Design review of the part built by this model. Coordinates are the model's own, in mm. A direction names the side the tool comes from. Coordinates: 2 decimals unless noted, no trailing zeros. Write each loop counter-clockwise with the first axis right and the second up, starting at its lowest first coordinate (ties: lowest second). Pieces come first, ordered by that corner, then holes. Notation, with made-up numbers: (2.25, 16.25) - (21.25, 16.25) arc R14 ccw to (21.25, 39.25) - close; hole circle Ø6 at (-39, 49.5). An arc over 180 degrees is marked (long way). Use a Markdown table: item, result.
from build123d import *

# Parameters (mm, degrees)
SKETCH1_W = 40
SKETCH1_H = 1
SKETCH2_W = 3
SKETCH2_H = 6


with BuildPart() as part:
    # Sketch1 → Base-Revolve (revolve)
    with BuildSketch(Plane.XY, mode=Mode.PRIVATE) as base_revolve_sk:
        with Locations((0, 4.5)):
            Rectangle(SKETCH1_W, SKETCH1_H)
    revolve(base_revolve_sk.sketch.rotate(Axis((-20, 0, 0), (1, 0, 0)), 90), axis=Axis((-20, 0, 0), (1, 0, 0)))

    # Sketch2 → Cut-for-GripLength (revolve, cut)
    with BuildSketch(Plane.XY):
        with Locations((-18.5, 3)):
            Rectangle(SKETCH2_W, SKETCH2_H)
        with Locations((18.5, 3)):
            Rectangle(SKETCH2_W, SKETCH2_H)
    revolve(axis=Axis((-30, 0, 0), (1, 0, 0)), mode=Mode.SUBTRACT)

    # Sketch3 → HeadTypeA (revolve)
    with BuildSketch(Plane.XY, mode=Mode.PRIVATE) as headtypea_sk:
        with BuildLine():
            Line((-19, 6), (-19, 7.5))
            Line((-19, 7.5), (-18, 7.5))
            Line((-18, 7.5), (-18, 6))
            ThreePointArc((-18, 6), (-17.707106781, 5.292893219), (-17, 5))
            Line((-17, 5), (-17, 4))
            ThreePointArc((-17, 4), (-18.414213562, 4.585786438), (-19, 6))
        make_face()
        with BuildLine():
            Line((19, 6), (19, 7.5))
            Line((19, 7.5), (18, 7.5))
            Line((18, 7.5), (18, 6))
            ThreePointArc((18, 6), (17.707106781, 5.292893219), (17, 5))
            Line((17, 5), (17, 4))
            ThreePointArc((17, 4), (18.414213562, 4.585786438), (19, 6))
        make_face()
    revolve(headtypea_sk.sketch.rotate(Axis((-20, 0, 0), (1, 0, 0)), 90), axis=Axis((-20, 0, 0), (1, 0, 0)))


solid = part.part
(1) Draft analysis for pull direction Z (two halves, no side actions). For faces 3 (the cylindrical face through (0.238, 3.905, -0.867)), 4 (the cylindrical face through (-18.493, -6.324, 4.032)), 5 (the flat face through (18, -6, 2)), state which applies: +Z half, -Z half, draft (parallel to the pull), parting line (faces both ways), or undercut.
Determined:
| item | result |
|---|---|
| face 3 | undercut |
| face 4 | parting line |
| face 5 | draft |
(2) Take a section at A-A on y = 0. Write out the cut boundary in (x, z), and give its area (3 significant figures).
Determined:
| item | result |
|---|---|
| outline | (-19, -7.5) - (-18, -7.5) - (-18, -6) arc R1 cw to (-17, -5) - (17, -5) arc R1 cw to (18, -6) - (18, -7.5) - (19, -7.5) - (19, -6) arc R2 ccw to (17, -4) - (-17, -4) arc R2 ccw to (-19, -6) - close; (-19, 6) arc R2 ccw to (-17, 4) - (17, 4) arc R2 ccw to (19, 6) - (19, 7.5) - (18, 7.5) - (18, 6) arc R1 cw to (17, 5) - (-17, 5) arc R1 cw to (-18, 6) - (-18, 7.5) - (-19, 7.5) - close |
| area | 83.4 mm2 |
(3) Take a section at C-C on x = -1. Write out the cut boundary in (y, z), and give its area (3 significant figures).
Determined:
| item | result |
|---|---|
| outline | circle Ø10 at (0, 0); hole circle Ø8 at (0, 0) |
| area | 28.3 mm2 |
(4) Take a section at D-D on y = -6.5. Write out the cut boundary in (x, z).
Determined:
| item | result |
|---|---|
| outline | (-19, -3.74) - (-18, -3.74) - (-18, 3.74) - (-19, 3.74) - close; (18, -3.74) - (19, -3.74) - (19, 3.74) - (18, 3.74) - close |
(5) For pin 1 (8 mm diameter, centred on y = -1, z = -4.5, fed in from +X); pin 2 (1.5 mm diameter, centred on x = -13, y = -2, fed in from -Z); pin 3 (6 mm diameter, centred on x = -14.5, z = -0.5, fed in from -Y); pin 4 (1 mm diameter, centred on x = -7.5, y = 0.5, fed in from +Z), all flat-tipped, find the tip position at first contact; note any pin that passes through.
Determined:
| item | result |
|---|---|
| pin 1 | x = 19 |
| pin 2 | z = -4.84 |
| pin 3 | y = -5.12 |
| pin 4 | z = 5 |
(6) Machinability: for faces 1 (the flat face through (-18, -6, 2)), 2 (the cylindrical face through (18.493, -6.324, 4.032)), which of the approach directions +Z, -Z, +X, -X, +Y, -Y give a long, thin tool a straight path to every point of the face, cutting with its end or side? Answer none if there is none.
Determined:
| item | result |
|---|---|
| face 1 | none |
| face 2 | +X, -X |
(7) For L1, parallel to Z at x = -6.5, y = -0.25; L2, parallel to X at y = -2.5, z = -6; L3, parallel to Y at x = 4, z = 0, list the stretches that pass through material, from the lowest coordinate up. Write a range as from..to.
Determined:
| item | result |
|---|---|
| L1 | -4.99..-3.99, 3.99..4.99 |
| L2 | -19..-18, 18..19 |
| L3 | -5..-4, 4..5 |
